```python
from build123d import *

# Parameters (mm, degrees)
CUT_EXTRUDE2_START = -7
SKETCH4_R          = 5
SKETCH4_R_2        = 3.9
CUT_EXTRUDE2_DEPTH = 7
SKETCH3_R          = 5
SKETCH3_R_2        = 3.9
CUT_EXTRUDE4_DEPTH = 12
CUT_EXTRUDE5_DEPTH = 5


with BuildPart() as part:
    # Sketch2 → Revolve1 (revolve)
    with BuildSketch(Plane(origin=(0, 0, 0), x_dir=(1, 0, 0), z_dir=(0, 1, 0))):
        Polygon((40, -5), (-40, -5), (-40, 0), (-30.049059985, 0), (-24.904700538, 0), (-23.75, -2), (-21.25, -2), (-20.095299462, 0), (-9.904700538, 0), (-8.75, -2), (-6.25, -2), (-5.095299462, 0), (5.095299462, 0), (6.25, -2), (8.75, -2), (9.904700538, 0), (20.095299462, 0), (21.25, -2), (23.75, -2), (24.904700538, 0), (30.049059985, 0), (40, 0), align=None)
    revolve(axis=Axis((40, 0, 5), (-1, 0, 0)))

    # Sketch4 → Cut-Extrude2 (cut)
    with BuildSketch(Plane.ZY.offset(40).offset(CUT_EXTRUDE2_START)):
        with Locations(Location((5, 0, 0), (0, 0, 180))):
            Circle(SKETCH4_R)
        with Locations((5, 0)):
            Circle(SKETCH4_R_2, mode=Mode.SUBTRACT)
    extrude(amount=CUT_EXTRUDE2_DEPTH, mode=Mode.SUBTRACT)

    # Sketch3 → Cut-Extrude4 (cut)
    with BuildSketch(Plane(origin=(40, 0, 0), x_dir=(0, 0, -1), z_dir=(1, 0, 0))):
        with Locations((-5, 0)):
            Circle(SKETCH3_R)
        with Locations(Location((-5, 0, 0), (0, 0, 180))):
            Circle(SKETCH3_R_2, mode=Mode.SUBTRACT)
    extrude(amount=-CUT_EXTRUDE4_DEPTH, mode=Mode.SUBTRACT)

    # Sketch5 → Cut-Extrude5 (cut)
    with BuildSketch(Plane(origin=(40, 0, 0), x_dir=(0, 0, -1), z_dir=(1, 0, 0))):
        with BuildLine():
            Line((-8.421971662, 1.870858078), (-1.578028338, 1.870858078))
            ThreePointArc((-1.578028338, 1.870858078), (-5, 3.9), (-8.421971662, 1.870858078))
        make_face()
    extrude(amount=-CUT_EXTRUDE5_DEPTH, mode=Mode.SUBTRACT)


solid = part.part
```
Here's how the part is built. I have some questions about the finished solid (model axes, mm). A direction names the side the tool comes from. Coordinates: 2 decimals unless noted, no trailing zeros. Order: outer loops, then holes, each group sorted by start corner. A loop starts at its lowest first (then second) coordinate and runs counter-clockwise, first axis right, second up.
1) We'd pull the mould along X, two halves only. Please class faces 4 (the face through (35, 3, 5)), 5 (the face through (-33, 3, 2)), 6 (the face through (7.52, -0.9, 2.14)): +X half, -X half, draft (parallel to the pull), parting line (faces both ways), or undercut.
2) I need wall thicknesses on line 1 (X direction, y = 0.75, z = 8); line 2 (X direction, y = -2.25, z = 1); line 3 (Y direction, x = 33, z = 2.5). Which ranges of each line are inside material? Lowest first, please.
3) Which directions (+Z, -Z, +X, -X, +Y, -Y) give clear straight access to the entire face, cutting with the end or side of a thin tool? Please do faces 1 (the face through (-29.01, -1.5, 0.23)), 2 (the face through (22.52, -0.9, 2.14)), 3 (the face through (-36.45, 1.17, 8.72)).
4) Will these pins go through, and if not, where does the flat tip stop? pin 1 (1 mm diameter, centred on x = -3, z = 2, fed in from -Y); pin 2 (1.5 mm diameter, centred on x = 37.5, z = 6.5, fed in from +Y); pin 3 (1.6 mm diameter, centred on y = 3.5, z = 3.5, fed in from +X).
5) Imagine slicing it at A-A on x = -23. List the corners of the cut face in (y, z) for me.
Response values:
1. face 4: +X half
1. face 5: -X half
1. face 6: undercut
2. line 1: x = -40 to -23.8, -21.2 to -8.8, -6.2 to 6.2, 8.8 to 21.2, 23.8 to 40
2. line 2: x = -33 to -24.67, -20.33 to -9.67, -5.33 to 5.33, 9.67 to 20.33, 24.67 to 28
2. line 3: y = -2.99 to 2.99
3. face 1: +X, -X
3. face 2: none
3. face 3: -X
4. pin 1: stops at y = -4.33
4. pin 2: stops at y = 1.87
4. pin 3: stops at x = 35
5. outline: circle Ø6 at (0, 5)
